The listing builds one solid part. Answer for the finished solid, in the listing's coordinates (mm). Face numbers are marked on the shaded views. Round coordinates to 2 decimals unless told otherwise and drop trailing zeros. Write each loop counter-clockwise with the first axis right and the second up, starting at its lowest first coordinate (ties: lowest second). Pieces come first, ordered by that corner, then holes. Notation, with made-up numbers: (-39, -34.75) - (8, -34.75) arc R17 ccw to (8, -8.75) - close; hole circle Ø8 at (16, 57). An arc over 180 degrees is marked (long way). Return JSON: item names as keys, results as strings. Group by question number.
from build123d import *

# Parameters (mm, degrees)
BOSS_EXTRUDE1_DEPTH = 40.64
SKETCH2_R           = 2.0193
CUT_EXTRUDE1_DEPTH  = 82.856729921


with BuildPart() as part:
    # Sketch1 → Boss-Extrude1 (new, symmetric)
    with BuildSketch(Plane.XY):
        Polygon((0, 7.332348419), (-6.35, 3.666174209), (-6.35, -3.666174209), (0, -7.332348419), (6.35, -3.666174209), (6.35, 3.666174209), align=None)
    extrude(amount=BOSS_EXTRUDE1_DEPTH, both=True)

    # Sketch2 → Cut-Extrude1 (cut, through all)
    with BuildSketch(Plane(origin=(0, 0, -40.64), x_dir=(-1, 0, 0), z_dir=(0, 0, -1))):
        Circle(SKETCH2_R)
    extrude(amount=-CUT_EXTRUDE1_DEPTH, mode=Mode.SUBTRACT)


solid = part.part
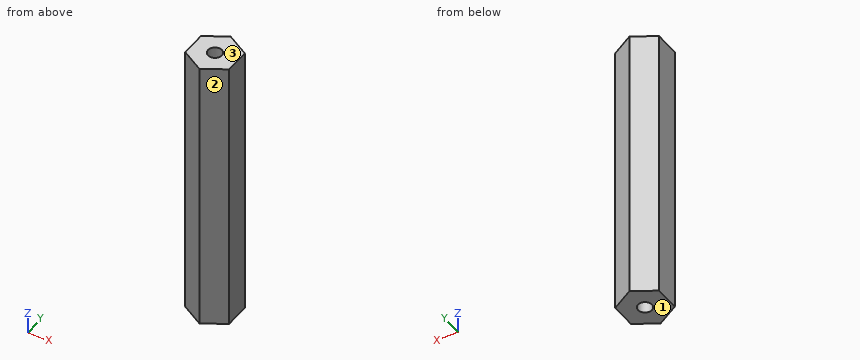
(1) Find section A-A (y = 0). Write down the section's boundary in (x, z), plus the area to 3 significant figures.
(2) Determine the mould class of the marked faces 1, 2 and 3 for opening direction Z: +Z half, -Z half, draft (parallel to the pull), parting line (faces both ways), or undercut.
(3) Flat-ended cylindrical pins translate along their axes: pin 1 (6 mm diameter, centred on y = 5, z = 28.5, fed in from +X); pin 2 (3 mm diameter, centred on x = -4.5, z = 10.5, fed in from -Y); pin 3 (3 mm diameter, centred on x = 3.5, z = 15, fed in from -Y); pin 4 (5 mm diameter, centred on x = -4, z = -28, fed in from +Y). Find the tip coordinate at first contact, or state that the pin passes through.
(4) Find section D-D (y = 5.75). Write down the section's boundary in (x, z), plus the area to 3 significant figures.
(5) Find section B-B (z = 32.5). Write down the section's boundary in (x, y).
(6) Consider line 1 (Y direction, x = 0, z = -10.5); line 2 (X direction, y = -0.25, z = -0.5); line 3 (X direction, y = 1.5, z = 34). Determine where each line is inside the solid, lowest interval first.
(7) Find section C-C (x = -3.5). Write down the section's boundary in (y, z).
Check sheet entries:
{
 "1": {"outline": "(-6.35, -40.64) - (-2.02, -40.64) - (-2.02, 40.64) - (-6.35, 40.64) - close; (2.02, -40.64) - (6.35, -40.64) - (6.35, 40.64) - (2.02, 40.64) - close", "area": "704 mm^2"},
 "2": {"face 1": "-Z half", "face 2": "draft", "face 3": "+Z half"},
 "3": {"pin 1": "stops at x = 6.35", "pin 2": "stops at y = -5.6", "pin 3": "stops at y = -6.18", "pin 4": "stops at y = 6.47"},
 "4": {"outline": "(-2.74, -40.64) - (2.74, -40.64) - (2.74, 40.64) - (-2.74, 40.64) - close", "area": "446 mm^2"},
 "5": {"outline": "(-6.35, -3.67) - (0, -7.33) - (6.35, -3.67) - (6.35, 3.67) - (0, 7.33) - (-6.35, 3.67) - close; hole circle Ø4.04 at (0, 0)"},
 "6": {"line 1": "y = -7.33 to -2.02, 2.02 to 7.33", "line 2": "x = -6.35 to -2, 2 to 6.35", "line 3": "x = -6.35 to -1.35, 1.35 to 6.35"},
 "7": {"outline": "(-5.31, -40.64) - (5.31, -40.64) - (5.31, 40.64) - (-5.31, 40.64) - close"}
}
